```python
from build123d import *

# Parameters (mm, degrees)
SKETCH1_R           = 1.5
BOSS_EXTRUDE1_DEPTH = 3


with BuildPart() as part:
    # Sketch1 → Boss-Extrude1 (new body)
    with BuildSketch(Plane(origin=(0, 0, 0), x_dir=(1, 0, 0), z_dir=(0, 1, 0))):
        with BuildLine():
            Line((0, -5), (23.998875872, -5))
            ThreePointArc((23.998875872, -5), (24.467345461, -4.883479623), (24.826642543, -4.561072489))
            Line((24.826642543, -4.561072489), (28.564941326, 0.954149161))
            ThreePointArc((28.564941326, 0.954149161), (28.766036178, 1.172359953), (29.022312673, 1.321950886))
            Line((29.022312673, 1.321950886), (40.929553216, 6.070049343))
            Line((40.929553216, 6.070049343), (45.451842333, 3.660227249))
            Line((45.451842333, 3.660227249), (46.37900311, 2.898073771))
            Line((46.37900311, 2.898073771), (47.144586244, 3.829406729))
            Line((47.144586244, 3.829406729), (48.06174016, 3.086958957))
            Line((48.06174016, 3.086958957), (48.804187932, 4.004112872))
            Line((48.804187932, 4.004112872), (49.721341848, 3.2616651))
            Line((49.721341848, 3.2616651), (50.46378962, 4.178819016))
            Line((50.46378962, 4.178819016), (51.380943536, 3.436371244))
            Line((51.380943536, 3.436371244), (52.123391308, 4.35352516))
            Line((52.123391308, 4.35352516), (53.040545224, 3.611077387))
            Line((53.040545224, 3.611077387), (53.782992996, 4.528231303))
            Line((53.782992996, 4.528231303), (54.700146912, 3.785783531))
            Line((54.700146912, 3.785783531), (55.442594685, 4.702937447))
            Line((55.442594685, 4.702937447), (56.34448506, 3.957791721))
            Line((56.34448506, 3.957791721), (57.05438411, 4.868693049))
            Line((57.05438411, 4.868693049), (51.831402108, 12.774604725))
            Line((51.831402108, 12.774604725), (46.024183924, 15.419882568))
            ThreePointArc((46.024183924, 15.419882568), (45.628323444, 15.509674561), (45.229386093, 15.434727162))
            Line((45.229386093, 15.434727162), (20.032711481, 5.075121772))
            ThreePointArc((20.032711481, 5.075121772), (19.846254378, 5.018960187), (19.652448068, 5))
            Line((19.652448068, 5), (0, 5))
            ThreePointArc((0, 5), (-5, 0), (0, -5))
        make_face()
        with Locations(Location((0, 0, 0), (0, 0, 270))):
            Circle(SKETCH1_R, mode=Mode.SUBTRACT)
        with Locations(Location((22, 0, 0), (0, 0, 270))):
            Circle(SKETCH1_R, mode=Mode.SUBTRACT)
    extrude(amount=BOSS_EXTRUDE1_DEPTH)


solid = part.part
```
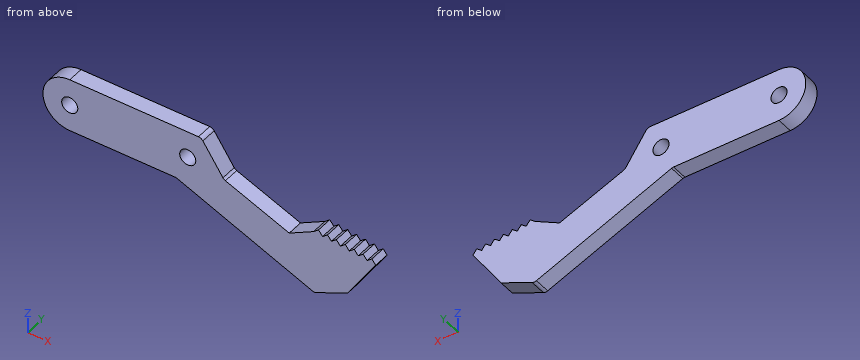
Model file for the job. Use its own axes, mm. Coordinates: 2 decimals unless noted, no trailing zeros. Order: outer loops, then holes, each group sorted by start corner. A loop starts at its lowest first (then second) coordinate and runs counter-clockwise, first axis right, second up. Notation, with made-up numbers: M 21,51 L 40,51 A14 cw 40,76 Z; hole C -24,-34 d4. An arc over 180 degrees is marked long. Answer as CSV lines item,"result".
(1) Band-saw the part on C-C, the plane z = 0. List the corners of the cut face in (x, y).
Geometry says:
outline,"M -5,0 L -1.5,0 L -1.5,3 L -5,3 Z; M 1.5,0 L 20.5,0 L 20.5,3 L 1.5,3 Z; M 23.5,0 L 27.92,0 L 27.92,3 L 23.5,3 Z"
(2) Band-saw the part on D-D, the plane x = 34. List the corners of the cut face in (y, z).
Geometry says:
outline,"M 0,-10.82 L 3,-10.82 L 3,-3.31 L 0,-3.31 Z"
(3) Wall check: line 1 along X through (y, z) = (1.95, 0); line 2 along Z through (x, y) = (15, 1.15); line 3 along X through (y, z) = (0.4, 2.25). Give the ranges that are in metal, low to high.
Geometry says:
line 1,"x = -5 to -1.5, 1.5 to 20.5, 23.5 to 27.92"
line 2,"z = -5 to 5"
line 3,"x = -4.47 to 26.39"
(4) Band-saw the part on B-B, the plane x = 22. List the corners of the cut face in (y, z), then the cut area to 3 significant figures.
Geometry says:
outline,"M 0,-5.88 L 3,-5.88 L 3,-1.5 L 0,-1.5 Z; M 0,1.5 L 3,1.5 L 3,5 L 0,5 Z"
area,"23.7 mm2"
(5) Flat gauge pin, fed straight in: pin 1 (2.5 mm diameter, centred on x = 22, z = 0, fed in from +Y). Where does the tip first touch, or does it go through?
Geometry says:
pin 1,"passes through"
(6) Band-saw the part on A-A, the plane y = 2.4. State how many separate pieces and enclosed holes the cut face has, then the cut area to 3 significant figures.
Geometry says:
separate pieces,"1"
enclosed holes,"2"
area,"544 mm2"
